Could you check a few things on this model? Use its own coordinates, in mm. A direction names the side the tool comes from. Round coordinates to 2 decimals unless told otherwise and drop trailing zeros. Loops run counter-clockwise (first coordinate to the right, second up) from the corner with the lowest first, then second, coordinate; pieces in that order, holes last. Notation, with made-up numbers: (-13, 79.25) -> (7, 79.25) arc R19 cw to (7, 86.25) -> close; hole circle Ø2 at (36, 25.5). An arc over 180 degrees is marked (long way). One line per item, written item: value.
Autodesk Inventor part; units mm, degrees
ref_plane "YZ Plane" through (0, 0, 0) normal (1, 0, 0) x (0, 1, 0)
ref_plane "XZ Plane" through (0, 0, 0) normal (0, 1, 0) x (-1, 0, 0)
ref_plane "XY Plane" through (0, 0, 0) normal (0, 0, 1) x (1, 0, 0)
sketch "Sketch1" plane through (0, 0, 0) normal (0, 1, 0) x (-1, 0, 0)
  line L0 (75, -0.4496) -> (0, -0.4496)
  line L1 (-21.1396, -9.0893) -> (-21.1396, -49.0893)
  line L2 (96.1396, -49.0893) -> (96.1396, -9.0893)
  circle A0 centre (72.69, -51.8993) radius 1.55
  circle A1 centre (2.31, -51.8993) radius 1.55
  circle A2 centre (72.69, -6.8993) radius 1.55
  circle A3 centre (2.31, -6.8993) radius 1.55
  arc A4 (-6, -7.8993) -> (-8, -5.8993) centre (-8, -7.8993) ccw
  line L3 (-14, -5.8993) -> (-8, -5.8993)
  arc A5 (-8, -10.8993) -> (-6, -8.8993) centre (-8, -8.8993) ccw
  line L4 (-6, -7.8993) -> (-6, -8.8993)
  arc A6 (-16, -8.8993) -> (-14, -10.8993) centre (-14, -8.8993) ccw
  line L5 (-16, -8.8993) -> (-16, -7.8993)
  arc A7 (-14, -5.8993) -> (-16, -7.8993) centre (-14, -7.8993) ccw
  arc A8 (89, -10.8993) -> (91, -8.8993) centre (89, -8.8993) ccw
  line L6 (91, -7.8993) -> (91, -8.8993)
  arc A9 (81, -8.8993) -> (83, -10.8993) centre (83, -8.8993) ccw
  line L7 (81, -8.8993) -> (81, -7.8993)
  arc A10 (91, -7.8993) -> (89, -5.8993) centre (89, -7.8993) ccw
  line L8 (83, -5.8993) -> (89, -5.8993)
  arc A11 (83, -5.8993) -> (81, -7.8993) centre (83, -7.8993) ccw
  arc A12 (2.2291, -16.0132) -> (-0.69, -17.7895) centre (1.31, -17.7895) ccw
  line L9 (-0.69, -40.389) -> (-0.69, -17.7895)
  arc A13 (24.0671, -30.8656) -> (24.0671, -27.313) centre (23.148, -29.0893) ccw
  line L10 (2.2291, -16.0132) -> (24.0671, -27.313)
  arc A14 (-0.69, -40.389) -> (2.2291, -42.1653) centre (1.31, -40.389) ccw
  line L11 (24.0671, -30.8656) -> (2.2291, -42.1653)
  arc A15 (23.6713, -40.2421) -> (24.4379, -44.0893) centre (24.4379, -42.0893) ccw
  line L12 (23.6713, -40.2421) -> (36.7334, -34.821)
  arc A16 (50.5621, -44.0893) -> (51.3287, -40.2421) centre (50.5621, -42.0893) ccw
  line L13 (38.2666, -34.821) -> (51.3287, -40.2421)
  arc A17 (38.2666, -34.821) -> (36.7334, -34.821) centre (37.5, -36.6682) ccw
  arc A18 (50.9329, -27.313) -> (50.9329, -30.8656) centre (51.852, -29.0893) ccw
  line L14 (50.9329, -27.313) -> (72.7709, -16.0132)
  arc A19 (75.69, -17.7895) -> (72.7709, -16.0132) centre (73.69, -17.7895) ccw
  line L15 (75.69, -17.7895) -> (75.69, -40.389)
  arc A20 (72.7709, -42.1653) -> (75.69, -40.389) centre (73.69, -40.389) ccw
  arc A21 (36.7334, -23.3576) -> (38.2666, -23.3576) centre (37.5, -21.5104) ccw
  line L16 (51.3287, -17.9365) -> (38.2666, -23.3576)
  arc A22 (51.3287, -17.9365) -> (50.5621, -14.0893) centre (50.5621, -16.0893) ccw
  line L17 (24.4379, -14.0893) -> (50.5621, -14.0893)
  arc A23 (24.4379, -14.0893) -> (23.6713, -17.9365) centre (24.4379, -16.0893) ccw
  line L18 (36.7334, -23.3576) -> (23.6713, -17.9365)
  line L19 (89, -10.8993) -> (83, -10.8993)
  line L20 (-8, -10.8993) -> (-14, -10.8993)
  circle A24 centre (-30.6843, -41.5893) radius 1.55
  circle A25 centre (105.6843, -41.5893) radius 1.55
  circle A26 centre (-30.6843, -16.5893) radius 1.55
  circle A27 centre (105.6843, -16.5893) radius 1.55
  line L21 (72.7709, -42.1653) -> (50.9329, -30.8656)
  line L22 (50.5621, -44.0893) -> (24.4379, -44.0893)
  arc A28 (-21, -55.0893) -> (-19, -57.0893) centre (-19, -55.0893) ccw
  line L23 (-19, -57.0893) -> (94, -57.0893)
  arc A29 (94, -57.0893) -> (96, -55.0893) centre (94, -55.0893) ccw
  line L24 (96, -50.5893) -> (96, -55.0893)
  arc A30 (96, -2.8993) -> (94, -0.8993) centre (94, -2.8993) ccw
  line L25 (94, -0.8993) -> (76.5, -0.8993)
  arc A31 (-19, -0.8993) -> (-21, -2.8993) centre (-19, -2.8993) ccw
  line L26 (-1.5, -0.8993) -> (-19, -0.8993)
  line L27 (96, -2.8993) -> (96, -7.5893)
  line L28 (-1.5, -1.6493) -> (-1.5, -0.8993)
  arc A32 (113.7793, -49.0893) -> (114.7793, -48.0893) centre (113.7793, -48.0893) ccw
  line L29 (114.7793, -10.0893) -> (114.7793, -48.0893)
  arc A33 (114.7793, -10.0893) -> (113.7793, -9.0893) centre (113.7793, -10.0893) ccw
  arc A34 (75, 21.19) -> (74, 22.19) centre (74, 21.19) ccw
  line L30 (1, 22.19) -> (74, 22.19)
  arc A35 (-39.7793, -48.0893) -> (-38.7793, -49.0893) centre (-38.7793, -48.0893) ccw
  arc A36 (-38.7793, -9.0893) -> (-39.7793, -10.0893) centre (-38.7793, -10.0893) ccw
  line L31 (-38.7793, -9.0893) -> (-19.94, -9.0893)
  arc A37 (1, 22.19) -> (0, 21.19) centre (1, 21.19) ccw
  line L32 (113.7793, -49.0893) -> (94.94, -49.0893)
  line L33 (-39.7793, -48.0893) -> (-39.7793, -10.0893)
  line L34 (96, -50.5893) -> (94.94, -50.5893)
  line L35 (94.94, -50.5893) -> (94.94, -49.0893)
  line L36 (94.94, -7.5893) -> (96, -7.5893)
  line L37 (94.94, -9.0893) -> (113.7793, -9.0893)
  line L38 (94.94, -9.0893) -> (94.94, -7.5893)
  line L39 (-21, -7.5893) -> (-19.94, -7.5893)
  line L40 (-19.94, -7.5893) -> (-19.94, -9.0893)
  line L41 (-21, -7.5893) -> (-21, -2.8993)
  line L42 (-19.94, -50.5893) -> (-21, -50.5893)
  line L43 (-19.94, -49.0893) -> (-38.7793, -49.0893)
  line L44 (-19.94, -49.0893) -> (-19.94, -50.5893)
  line L45 (-21, -55.0893) -> (-21, -50.5893)
  line L46 (75, 21.19) -> (75, -1.6493)
  line L47 (0, -1.6493) -> (0, 21.19)
  line L48 (0, -1.6493) -> (-1.5, -1.6493)
  line L49 (76.5, -0.8993) -> (76.5, -1.6493)
  line L50 (76.5, -1.6493) -> (75, -1.6493)
  line L51 (96.5893, -9.0893) -> (96.5893, -49.0893)
  line L52 (-21.5893, -49.0893) -> (-21.5893, -9.0893)
  line L53 (95.69, -49.0893) -> (95.69, -9.0893)
  line L54 (-20.69, -9.0893) -> (-20.69, -49.0893)
  line L55 (75, -0.8993) -> (0, -0.8993)
  line L56 (0, 0) -> (75, 0)
extrude "Extrusion1" add sketch "Sketch1" against normal blind 1.5
properties part number "body_back_frame"
(1) Imagine slicing it at C-C on x = -79.5. Write out the boundary of the cut face in (y, z), then the cut area to 3 significant figures.
Results below:
outline: (-1.5, -57.09) -> (0, -57.09) -> (0, -0.9) -> (-1.5, -0.9) -> close
area: 84.3 mm²
(2) We'd pull the mould along Z, two halves only. Please class faces 3 (the face through (-36, 0, -26)), 4 (the face through (-62, -0.74, -36.59)), 5 (the face through (-30.11, -0.74, -37.57)): +Z half, -Z half, draft (parallel to the pull), parting line (faces both ways), or undercut.
Results below:
face 3: draft
face 4: undercut
face 5: undercut
(3) Imagine slicing it at A-A on x = -20. Write out the boundary of the cut face in (y, z).
Results below:
outline: (-1.5, -57.09) -> (0, -57.09) -> (0, -32.97) -> (-1.5, -32.97) -> close; (-1.5, -25.21) -> (0, -25.21) -> (0, 22.19) -> (-1.5, 22.19) -> close
(4) On a 3-axis mill with a long thin cutter (end or side, diameter ignored), from which of +Z, -Z, +X, -X, +Y, -Y can I reach the whole of each face in a straight line? I mean faces 1 (the face through (-12.995, -0.74, -21.584)), 2 (the face through (-36, -1.5, -26)). Say none if no direction works.
Results below:
face 1: +Y, -Y
face 2: +Z, -Z, +X, -X, -Y
(5) Imagine slicing it at B-B on y = -1.15. Give the number of separate pieces and of enclosed holes in the cut face, then the cut area to 3 significant figures.
Results below:
separate pieces: 1
enclosed holes: 14
area: 8,450 mm²
(6) For pin 1 Ø0.6 at (y, z) = (-0.5, -1.5) entering from -X; pin 2 Ø1.9 at (x, z) = (30.68, -41.59) entering from -Y; pin 3 Ø3 at (x, z) = (-76.5, -8.5) entering from +Y; pin 4 Ø0.6 at (y, z) = (-1, -1.5) entering from +X, each with a flat end and sliding along its axis, tell me the tip position at first contact or that it passes through.
Results below:
pin 1: stops at x = -95.67
pin 2: passes through
pin 3: stops at y = 0
pin 4: stops at x = 20.67
(7) Please list where these lines run through material, in increasing order: L1, parallel to Z at x = 14, y = -1.3; L2, parallel to X at y = -1.1, z = -25; L3, parallel to X at y = -1.3, z = -35.
Results below:
L1: z = -57.09 to -10.9, -5.9 to -0.9
L2: x = -114.78 to -75.69, -55.4 to -19.6, 0.69 to 39.78
L3: x = -114.78 to -75.69, -58.92 to -38.7, -36.3 to -16.08, 0.69 to 39.78
